Build history of the part. All positions in model axes, mm. Round coordinates to 2 decimals unless told otherwise and drop trailing zeros. Write each loop counter-clockwise with the first axis right and the second up, starting at its lowest first coordinate (ties: lowest second). Pieces come first, ordered by that corner, then holes. Notation, with made-up numbers: M 55,1.5 L 111,1.5 A19 cw 111,17.5 Z; hole C 15.25,-39.75 d8. An arc over 180 degrees is marked long. Write item = value, one per line.
from build123d import *

# Parameters (mm, degrees)
F0_R     = 60
F1_DEPTH = 25
F2_DEPTH = 25
F3_DEPTH = 37
F4_R     = 15
F5_R     = 45
F6_DEPTH = 25


with BuildPart() as f1:
    # F0 (on Front) → F1 (new body)
    with BuildSketch(Plane.XZ):
        with Locations((20.5037463456, 3.3097660635)):
            Circle(F0_R)
    extrude(amount=F1_DEPTH)

    # F2 (add): faces of the model
    f2_faces = [f1.faces().sort_by_distance(p)[0] for p in [
        (20.5037463456, -25, 3.3097660635),
        (20.5037463456, 0, 3.3097660635),
    ]]
    extrude(f2_faces, amount=F2_DEPTH, dir=(0, -1, 0))

    # F3 (intersect): a face of the model
    f3_faces = [f1.faces().sort_by_distance(p)[0] for p in [
        (20.5037463456, -50, 3.3097660635),
    ]]
    extrude(f3_faces, amount=-F3_DEPTH, mode=Mode.INTERSECT)

    # F4
    f4_edges = [f1.edges().sort_by_distance(p)[0] for p in [
        (-39.496254, -50, 3.309766),
    ]]
    fillet(f4_edges, radius=F4_R)

    # F5 (on face) → F6 (cut)
    with BuildSketch(Plane.XZ.offset(50)):
        with Locations((20.5037463456, 3.3097660635)):
            Circle(F5_R)
    extrude(amount=-F6_DEPTH, mode=Mode.SUBTRACT)


solid = f1.part
1. Band-saw the part on A-A (y = -47). List the corners of the cut face in (x, z).
Responses:
outline = C 20.5,3.31 d108; hole C 20.5,3.31 d90
2. Flat gauge pins, fed straight in: pin 1 (2 mm diameter, centred on y = -21, z = 40, fed in from -X); pin 2 (6 mm diameter, centred on y = -46, z = 21, fed in from +X); pin 3 (1 mm diameter, centred on x = -26.5, z = -26, fed in from -Y). Where does each tip first touch, or does it go through?
Responses:
pin_1 = -27.73
pin_2 = 75.62
pin_3 = -46.27
3. Mould opens along X. For faces 1 (the face through (20, -25, 4)), 2 (the face through (20, -13, 4)), 3 (the face through (-23.72, -24.15, 43.86)) say: pulls with the +X half, pulls with the -X half, needs draft (parallel to the pull), parting line crosses it, or undercut.
Responses:
face_1 = undercut
face_2 = needs draft
face_3 = parting line crosses it
4. Probe probe 1 along Y at (x, z) = (14, -36.5); probe 2 along Z at (x, y) = (19.5, -43.5); probe 3 along Z at (x, y) = (55, -35). List the from-to ranges inside material, lowest first.
Responses:
probe_1 = -25 to -13
probe_2 = -54.04 to -41.68, 48.3 to 60.66
probe_3 = -45.78 to -25.59, 32.21 to 52.4
